Could you check a few things on this model? Use its own coordinates, in mm. Coordinates: 2 decimals unless noted, no trailing zeros. Loops run counter-clockwise (first coordinate to the right, second up) from the corner with the lowest first, then second, coordinate; pieces in that order, holes last. Notation, with made-up numbers: M 88,-25.5 L 105,-25.5 A22 cw 105,-9.5 Z; hole C 43.5,24 d10. An arc over 180 degrees is marked long. Write each question's results on one line, items separated by ' | '.
```python
from build123d import *

# Parameters (mm, degrees)
BOSS_EXTRUDE1_DEPTH = 4.3


with BuildPart() as part:
    # Sketch4 → Boss-Extrude1 (new body)
    with BuildSketch(Plane(origin=(0, 0, 0), x_dir=(1, 0, 0), z_dir=(0, 1, 0))):
        with BuildLine():
            Line((47.736880922, -13.610395438), (47.736880922, -10.518490221))
            Line((47.736880922, -10.518490221), (-2.263119078, -11.062941575))
            Line((-2.263119078, -11.062941575), (-31.934689225, -41.387814618))
            Line((-31.934689225, -41.387814618), (-143.77908283, -42.60569125))
            Line((-143.77908283, -42.60569125), (-143.77908283, -48.60569125))
            Line((-143.77908283, -48.60569125), (-148.07908283, -48.60569125))
            Line((-148.07908283, -48.60569125), (-148.07908283, -58.60569125))
            Line((-148.07908283, -58.60569125), (-143.77908283, -58.60569125))
            Line((-143.77908283, -58.60569125), (-143.77908283, -84.761876256))
            Line((-143.77908283, -84.761876256), (-148.07908283, -84.761876256))
            Line((-148.07908283, -84.761876256), (-148.07908283, -94.761876256))
            Line((-148.07908283, -94.761876256), (-143.77908283, -94.761876256))
            Line((-143.77908283, -94.761876256), (-143.77908283, -100.761876256))
            Line((-143.77908283, -100.761876256), (96.389605884, -98.512277012))
            ThreePointArc((96.389605884, -98.512277012), (109.998414099, -89.747620618), (123.769012787, -98.255821046))
            Line((123.769012787, -98.255821046), (143.77908283, -98.068391791))
            Line((143.77908283, -98.068391791), (143.77908283, -92.068391791))
            Line((143.77908283, -92.068391791), (148.07908283, -92.068391791))
            Line((148.07908283, -92.068391791), (148.07908283, -80.068391791))
            Line((148.07908283, -80.068391791), (143.77908283, -80.068391791))
            Line((143.77908283, -80.068391791), (143.77908283, -34.269759798))
            Line((143.77908283, -34.269759798), (148.07908283, -34.269759798))
            Line((148.07908283, -34.269759798), (148.07908283, -22.269759798))
            Line((148.07908283, -22.269759798), (143.77908283, -22.269759798))
            Line((143.77908283, -22.269759798), (143.77908283, -16.269759798))
            Line((143.77908283, -16.269759798), (47.736880922, -13.610395438))
        make_face()
    extrude(amount=-BOSS_EXTRUDE1_DEPTH)


solid = part.part
```
(1) Imagine slicing it at C-C, the plane x = -43.5. List the corners of the cut face in (y, z) for me, and give its area (3 significant figures).
Reported:
outline: M -4.3,41.51 L 0,41.51 L 0,99.82 L -4.3,99.82 Z | area: 251 mm2
(2) If we mould it in two halves opening along X, with no side actions, what happens to faces 1 (the flat face through (-2, 0, 65)), 2 (the flat face through (-16.89, -2.12, 26.01)), 3 (the cylindrical face through (109.76, -2.12, 89.75))? For each: released by +X, released by -X, zero draft, split by the parting line, or undercut.
Reported:
face 1: zero draft | face 2: released by -X | face 3: undercut
(3) Please list where these lines run through material, in increasing order: probe 1 along X at (y, z) = (-3.75, 60); probe 2 along X at (y, z) = (-0.65, 92.5); probe 3 along Z at (x, y) = (100, -1.4). Write a range as from..to.
Reported:
probe 1: x = -143.78..143.78 | probe 2: x = -148.08..101.43, 118.85..143.78 | probe 3: z = 15.06..93.63
(4) Will these pins go through, and if not, where does the flat tip stop? P1, Ø2, axis at x = -146.5, y = -2, coming from the +Z side; P2, Ø1.3, axis at y = -2.5, z = 45.5, coming from the -X side; P3, Ø2.5, axis at y = -2.5, z = 11.5, coming from the +X side.
Reported:
P1: stops at z = 94.76 | P2: stops at x = -143.78 | P3: stops at x = 47.74
(5) Imagine slicing it at B-B, the plane z = 74. List the corners of the cut face in (x, y) for me.
Reported:
outline: M -143.78,-4.3 L 143.78,-4.3 L 143.78,0 L -143.78,0 Z
(6) Imagine slicing it at A-A, the plane y = -1.7. List the corners of the cut face in (x, z) for me, and give its area (3 significant figures).
Reported:
outline: M -148.08,48.61 L -143.78,48.61 L -143.78,42.61 L -31.93,41.39 L -2.26,11.06 L 47.74,10.52 L 47.74,13.61 L 143.78,16.27 L 143.78,22.27 L 148.08,22.27 L 148.08,34.27 L 143.78,34.27 L 143.78,80.07 L 148.08,80.07 L 148.08,92.07 L 143.78,92.07 L 143.78,98.07 L 123.77,98.26 A15.17 cw 96.39,98.51 L -143.78,100.76 L -143.78,94.76 L -148.08,94.76 L -148.08,84.76 L -143.78,84.76 L -143.78,58.61 L -148.08,58.61 Z | area: 21,200 mm2
